Could you check a few things on this model? Use its own coordinates, in mm. A direction names the side the tool comes from. Give positions to 0.01 mm unless a question says otherwise; leave off trailing zeros. Write each loop counter-clockwise with the first axis right and the second up, starting at its lowest first coordinate (ties: lowest second). Pieces come first, ordered by that corner, then holes. Notation, with made-up numbers: (25, -9.5) - (60, -9.5) arc R17 ccw to (60, 8.5) - close; hole circle Ø5 at (64, -8). An arc over 180 degrees is marked (long way). Answer as CSV lines item,"result". Start each with the question number.
Q1. On a 3-axis mill with a long thin cutter (end or side, diameter ignored), from which of +Z, -Z, +X, -X, +Y, -Y can I reach the whole of each face in a straight line? I mean faces 1 (the face through (37.691, 26.635, 2.504)), 2 (the face through (205, 14, 0)). Say none if no direction works.
Q2. Will this pin go through, and if not, where does the flat tip stop? pin 1 Ø3 at (y, z) = (30.5, 4.5) entering from +X.
Q3. Imagine slicing it at A-A on z = 3.35. List the corners of the cut face in (x, y) for me (3 decimals).
Q4. Imagine slicing it at C-C on x = 45.5. List the corners of the cut face in (y, z) for me.
Q5. If I drill on line 1 along Y through (x, z) = (254, 1.95); line 2 along X through (y, z) = (35, 2.45); line 3 along X through (y, z) = (18.5, 3.1), over which ranges is the centre line in solid material (lowest first)?
Q6. Imagine slicing it at B-B on x = 141. List the corners of the cut face in (y, z) for me, and give its area (3 significant figures).
Q7. We'd pull the mould along X, two halves only. Please class faces 3 (the face through (386.375, 3.316, 2.504)), 4 (the face through (379.13, 26.79, 2.5)), 5 (the face through (30.598, 3.136, 2.504)), 6 (the face through (205, 14, 5.08)): pulls with the +X half, pulls with the -X half, needs draft (parallel to the pull), parting line crosses it, or undercut.
Autodesk Inventor part; units mm, degrees
ref_plane "YZ Plane" through (0, 0, 0) normal (1, 0, 0) x (0, 1, 0)
ref_plane "XZ Plane" through (0, 0, 0) normal (0, 1, 0) x (-1, 0, 0)
ref_plane "XY Plane" through (0, 0, 0) normal (0, 0, 1) x (1, 0, 0)
sketch "Sketch1" plane through (0, 0, 0) normal (0, 0, 1) x (1, 0, 0)
  line L0 (55.4931, -0.0207) -> (359.029, -0.0207)
  line L1 (208.28, -0.0207) -> (55.4931, -0.0207)
  line L2 (208.28, -0.0207) -> (359.029, -0.0207)
  line L3 (57.245, 23.9209) -> (359.029, 23.9209)
  line L4 (208.28, -0.0207) -> (359.029, -0.0207)
  line L5 (55.4931, -0.0207) -> (359.0367, -0.0207)
  line L6 (359.0367, 23.9209) -> (57.245, 23.9209)
  arc A0 (19.6495, 34.5513) -> (6.6543, 12.7528) centre (12.7, 23.9214) ccw
  arc A1 (19.138, 34.8687) -> (57.245, 23.9209) centre (57.245, 95.7161) ccw
  arc A2 (6.262, 12.9742) -> (55.4931, -0.0207) centre (55.4931, 99.7327) ccw
  arc A3 (409.6274, 12.7528) -> (396.6322, 34.5513) centre (403.5817, 23.9214) ccw
  arc A4 (359.0367, 23.9209) -> (397.1436, 34.8687) centre (359.0367, 95.7161) ccw
  arc A5 (360.7886, -0.0207) -> (410.0197, 12.9742) centre (360.7886, 99.7327) ccw
  line L7 (360.7886, -0.0207) -> (55.4931, -0.0207)
  point P0 (0, 0)
  point P1 (416.2817, 0)
extrude "Extrusion1" add sketch "Sketch1" along normal blind 5.08 contours A2 A0 A1 L3 L6 A4 A3 A5 L7 L5 L0
properties part number "bottomSkid"
Conclusion:
1,face 1,"+Z, -Z, +Y"
1,face 2,"-Z, +X, -X, +Y, -Y"
2,pin 1,"x = 415.22"
3,outline,"(6.654, 12.753) arc R99.754 ccw to (55.493, -0.021) - (360.789, -0.021) arc R99.753 ccw to (409.627, 12.753) arc R12.7 ccw (long way) to (397.144, 34.869) arc R71.794 cw to (359.037, 23.921) - (57.245, 23.921) arc R71.795 cw to (19.138, 34.869) arc R12.7 ccw (long way) to start"
4,outline,"(0.48, 0) - (24.89, 0) - (24.89, 5.08) - (0.48, 5.08) - close"
5,line 1,"-0.02 to 23.92"
5,line 2,"6.49 to 18.91, 397.37 to 409.79"
5,line 3,"1.22 to 415.07"
6,outline,"(-0.02, 0) - (23.92, 0) - (23.92, 5.08) - (-0.02, 5.08) - close"
6,area,"122 mm^2"
7,face 3,"pulls with the +X half"
7,face 4,"undercut"
7,face 5,"pulls with the -X half"
7,face 6,"needs draft"
